Read the model definition and answer for the solid it produces. Units are mm, in the model's axes. A direction names the side the tool comes from. Coordinates: 2 decimals unless noted, no trailing zeros. Write each loop counter-clockwise with the first axis right and the second up, starting at its lowest first coordinate (ties: lowest second). Pieces come first, ordered by that corner, then holes.
Item 1: Determine the mould class of faces 1 (the face through (-0.5, 6, -9.1)), 2 (the face through (12, 7, -19)), 3 (the face through (12, 0, -9)) for opening direction Y: released by +Y, released by -Y, zero draft, split by the parting line, or undercut.
Item 2: This flat-tipped pin is pushed along its axis until it touches: P1, Ø1, axis at x = 18, z = -14.5, coming from the +Y side. Where does it stop, or does it pass through?
Item 3: Section C-C (x = 23.75) is taken. Give the vertices of the cut face in (y, z).
Item 4: A tool of negligible diameter and unlimited length cuts with its end or side. For faces 4 (the face through (12, 7, -18)), 5 (the face through (-0.5, 8.5, -4)), 6 (the face through (26, 7, -9)), from which of +Z, -Z, +X, -X, +Y, -Y can it reach the whole face along a straight path? Write none if from no direction.
Item 5: Section D-D (y = 10) is taken. Give the vertices of the cut face in (x, z), then the cut area to 3 significant figures.
Item 6: Straight lines are drawn through the part: probe 1 along Z at (x, y) = (16.5, 7.75); probe 2 along X at (y, z) = (6, -17.75); probe 3 along Y at (x, z) = (22.75, -1.5). For each, find the intervals that lie inside material, in ascending order.
Item 7: Section B-B (z = -5) is taken. Give the vertices of the cut face in (x, y).
Item 8: Section A-A (y = 5.5) is taken. Give the vertices of the cut face in (x, z), then the cut area to 3 significant figures.
from build123d import *

# Parameters (mm, degrees)
CROQUIS1_W              = 27
CROQUIS1_H              = 20
CROQUIS1_W_2            = 25
CROQUIS1_H_2            = 18
SALIENTE_EXTRUIR1_DEPTH = 14
CROQUIS1_3_W            = 25
CROQUIS1_3_H            = 18
SALIENTE_EXTRUIR2_DEPTH = 1
CROQUIS2_W              = 5
CROQUIS2_H              = 5
CORTAR_EXTRUIR1_DEPTH   = 1


with BuildPart() as part:
    # Croquis1 → Saliente-Extruir1 (new body)
    with BuildSketch(Plane(origin=(0, 0, 0), x_dir=(1, 0, 0), z_dir=(0, 1, 0))):
        with Locations((12.5, 9)):
            Rectangle(CROQUIS1_W, CROQUIS1_H)
        with Locations((12.5, 9)):
            Rectangle(CROQUIS1_W_2, CROQUIS1_H_2, mode=Mode.SUBTRACT)
    extrude(amount=SALIENTE_EXTRUIR1_DEPTH)

    # Croquis1_3 → Saliente-Extruir2 (add)
    with BuildSketch(Plane(origin=(0, 0, 0), x_dir=(1, 0, 0), z_dir=(0, 1, 0))):
        with Locations((12.5, 9)):
            Rectangle(CROQUIS1_3_W, CROQUIS1_3_H)
    extrude(amount=SALIENTE_EXTRUIR2_DEPTH)

    # Croquis2 → Cortar-Extruir1 (cut)
    with BuildSketch(Plane.ZY.offset(1)):
        with Locations((-11.5, 8.5)):
            Rectangle(CROQUIS2_W, CROQUIS2_H)
        with Locations((-6.5, 8.5)):
            Rectangle(CROQUIS2_W, CROQUIS2_H)
    extrude(amount=-CORTAR_EXTRUIR1_DEPTH, mode=Mode.SUBTRACT)


solid = part.part
Established:
1. face 1: undercut
1. face 2: zero draft
1. face 3: released by -Y
2. P1: stops at y = 1
3. outline: (0, -19) - (14, -19) - (14, -18) - (1, -18) - (1, 0) - (14, 0) - (14, 1) - (0, 1) - close
4. face 4: +Y
4. face 5: -X
4. face 6: +Z, -Z, +X, +Y, -Y
5. outline: (-1, -19) - (26, -19) - (26, 1) - (-1, 1) - (-1, -4) - (0, -4) - (0, 0) - (25, 0) - (25, -18) - (0, -18) - (0, -14) - (-1, -14) - close
5. area: 80.0 mm2
6. probe 1: z = -19 to -18, 0 to 1
6. probe 2: x = -1 to 0, 25 to 26
6. probe 3: y = 0 to 1
7. outline: (-1, 0) - (26, 0) - (26, 14) - (25, 14) - (25, 1) - (0, 1) - (0, 6) - (-1, 6) - close; (-1, 11) - (0, 11) - (0, 14) - (-1, 14) - close
8. outline: (-1, -19) - (26, -19) - (26, 1) - (-1, 1) - close; hole (0, -18) - (25, -18) - (25, 0) - (0, 0) - close
8. area: 90.0 mm2
